from build123d import *

# Parameters (mm, degrees)
F0_R     = 45
F1_DEPTH = 15


# Not quite as in the source:
# - ends of sketch curves that miss each other by under 0.0002 mm in the source are joined


with BuildPart() as f1:
    # F0 (on Front) → F1 (new body)
    with BuildSketch(Plane.XZ):
        with BuildLine():
            Line((508.886889, 467.23394), (536.629649, 437.761061))
            ThreePointArc((536.629649, 437.761061), (757.5121515647, 538.3707556644), (915.8713779319, 722.3102730367))
            ThreePointArc((915.8713779319, 722.3102730367), (937.3750069367, 871.1241026292), (891.6662720762, 1014.3675090452))
            ThreePointArc((891.6662720762, 1014.3675090452), (857.8155387776, 1059.5076628094), (819.4482445104, 1100.877414496))
            ThreePointArc((819.4482445104, 1100.877414496), (817.2633574779, 1103.137500552), (815.2248101142, 1105.5304160912))
            ThreePointArc((815.2248101142, 1105.5304160912), (734.7474434458, 1114.8247485045), (724.8508240235, 1034.4192260182))
            ThreePointArc((724.8508240235, 1034.4192260182), (789.4425603105, 903.419496525), (799.5567075135, 757.7118249354))
            ThreePointArc((799.5567075135, 757.7118249354), (793.3301361175, 732.8130625575), (780.9710848276, 710.319232126))
            ThreePointArc((780.9710848276, 710.319232126), (657.7707545167, 574.4028574869), (508.886889, 467.23394))
        make_face()
        with Locations((860.37194, 943.574077)):
            Circle(F0_R, mode=Mode.SUBTRACT)
        with Locations((770.304035, 1069.636489)):
            Circle(F0_R, mode=Mode.SUBTRACT)
    extrude(amount=F1_DEPTH)


solid = f1.part
CAD build for the part. Positions are in the model's coordinates, mm. A direction names the side the tool comes from. Coordinates: 2 decimals unless noted, no trailing zeros. Write each loop counter-clockwise with the first axis right and the second up, starting at its lowest first coordinate (ties: lowest second). Pieces come first, ordered by that corner, then holes. Notation, with made-up numbers: (31, -32) - (71, -32) arc R13 cw to (71, -14) - close; hole circle Ø11 at (5.5, -29). An arc over 180 degrees is marked (long way). Use a Markdown table: item, result. Add a question column.
Item 1: 3-axis set-ups, long thin cutter, end or side, ignore diameter. For faces 4 (the face through (522.564, -7.395, 452.704)), 5 (the face through (659.69, -7.4, 576.12)): which of +Z, -Z, +X, -X, +Y, -Y reach the whole face in a straight line?
Item 2: Band-saw the part on C-C, the plane x = 883.5. Give the cut face in (y, z).
Item 3: Flat gauge pins, fed straight in: pin 1 (1 mm diameter, centred on x = 553.5, y = -8.5, fed in from -Z); pin 2 (5 mm diameter, centred on x = 586, y = -6.5, fed in from +Z); pin 3 (2 mm diameter, centred on x = 680.5, y = -6.5, fed in from +Z); pin 4 (10 mm diameter, centred on x = 684.5, z = 605, fed in from +Y). Where does each tip first touch, or does it go through?
Item 4: Band-saw the part on B-B, the plane y = -3. Give the cut face in (x, z).
Item 5: Band-saw the part on D-D, the plane z = 671. Give the cut face in (x, y).
Item 6: Mould opens along X. For faces 1 (the face through (827.21, -7.4, 973.99)), 2 (the face through (937.544, -7.395, 869.008)), 3 (the face through (735.74, -7.4, 1115.59)) say: pulls with the +X half, pulls with the -X half, needs draft (parallel to the pull), parting line crosses it, or undercut.
Item 7: Band-saw the part on A-A, the plane x = 774. Give the cut face in (y, z), and give its area (3 significant figures).
Item 8: Drill centre lines: L1, parallel to Z at x = 760, y = -9.5; L2, parallel to Z at x = 717.5, y = -11; L3, parallel to Z at x = 894.5, y = -1. Where is each one in solid material? Low to high. Write a range as from..to.
Numbers:
| question | item | result |
|---|---|---|
| 1 | face 4 | -Z, -X, +Y, -Y |
| 1 | face 5 | -X, +Y, -Y |
| 2 | outline | (-15, 669.44) - (0, 669.44) - (0, 904.97) - (-15, 904.97) - close; (-15, 982.18) - (0, 982.18) - (0, 1026.19) - (-15, 1026.19) - close |
| 3 | pin 1 | z = 441.52 |
| 3 | pin 2 | z = 518.59 |
| 3 | pin 3 | z = 596.41 |
| 3 | pin 4 | y = 0 |
| 4 | outline | (508.89, 467.23) - (536.63, 437.76) arc R565.49 ccw to (915.87, 722.31) arc R335.22 ccw to (891.67, 1014.37) arc R541.09 ccw to (819.45, 1100.88) arc R50 cw to (815.22, 1105.53) arc R57.5 ccw to (724.85, 1034.42) arc R378.06 cw to (799.56, 757.71) arc R100 cw to (780.97, 710.32) arc R872.95 cw to start; hole circle Ø90 at (770.3, 1069.64); hole circle Ø90 at (860.37, 943.57) |
| 5 | outline | (750.48, -15) - (884.58, -15) - (884.58, 0) - (750.48, 0) - close |
| 6 | face 1 | undercut |
| 6 | face 2 | pulls with the +X half |
| 6 | face 3 | parting line crosses it |
| 7 | outline | (-15, 551.22) - (0, 551.22) - (0, 700.91) - (-15, 700.91) - close; (-15, 948.91) - (0, 948.91) - (0, 1024.79) - (-15, 1024.79) - close; (-15, 1114.48) - (0, 1114.48) - (0, 1127.02) - (-15, 1127.02) - close |
| 7 | area | 3,570 mm2 |
| 8 | L1 | 540.25..682.79, 979.05..1025.83, 1113.44..1126.21 |
| 8 | L2 | 510.95..633.16, 1046.88..1092.4 |
| 8 | L3 | 685.98..914.24, 972.9..1009.49 |
